from build123d import *

# Parameters (mm, degrees)
CHAMFER_SIZE    = 1
SKETCH001_R     = 2.25
SKETCH001_R_2   = 1.95
POCKET_DEPTH    = 2
CHAMFER001_SIZE = 0.5
POCKET001_DEPTH = 3


with BuildPart() as part:
    # Sketch (on XZ_Plane of Origin) → Revolution (revolve)
    with BuildSketch(Plane.XZ):
        Polygon((0, 0), (29.6, 0), (29.6, 7.7), (23.5, 7.7), (23.5, 6.2), (0, 6.2), align=None)
    revolve(axis=Axis((0, 0, 0), (0, 0, 1)))

    # Chamfer
    chamfer_edges = [part.edges().sort_by_distance(p)[0] for p in [
        (-23.5, 0, 7.7),
    ]]
    chamfer(chamfer_edges, length=CHAMFER_SIZE)

    # Sketch001 (on XY_Plane of Origin) → Pocket (cut)
    with BuildSketch(Plane.XY):
        Circle(SKETCH001_R)
        with Locations((14, 0)):
            Circle(SKETCH001_R_2)
        with Locations((-14, 0)):
            Circle(SKETCH001_R_2)
    extrude(amount=POCKET_DEPTH, mode=Mode.SUBTRACT)

    # Chamfer001
    chamfer001_edges = [part.edges().sort_by_distance(p)[0] for p in [
        (-29.6, 0, 7.7),
        (-29.6, 0, 0),
    ]]
    chamfer(chamfer001_edges, length=CHAMFER001_SIZE)

    # Sketch002 (on XY_Plane of Origin) → Pocket001 (cut)
    with BuildSketch(Plane.XY):
        with BuildLine():
            ThreePointArc((2, -22.1), (0, -20.1), (-2, -22.1))
            Line((-2, -22.1), (-2, -31.1))
            ThreePointArc((-2, -31.1), (0, -33.1), (2, -31.1))
            Line((2, -22.1), (2, -31.1))
        make_face()
    extrude(amount=POCKET001_DEPTH, mode=Mode.SUBTRACT)


solid = part.part
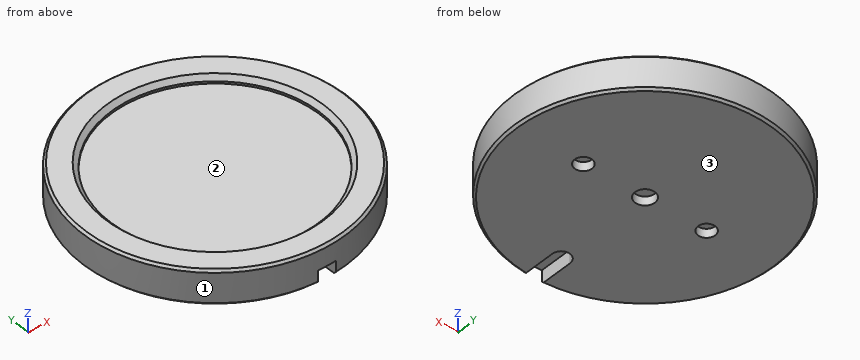
Geometry check sheet. Reference: the model listing, model coordinates, mm. Face numbers are marked on the shaded views. Round coordinates to 2 decimals unless told otherwise and drop trailing zeros. Write each loop counter-clockwise with the first axis right and the second up, starting at its lowest first coordinate (ties: lowest second). Pieces come first, ordered by that corner, then holes. Notation, with made-up numbers: (-1.5, 34.5) -> (54.5, 34.5) arc R16 cw to (54.5, 44.5) -> close; hole circle Ø4 at (-34.75, 4.25). An arc over 180 degrees is marked (long way). One line per item, written item: value. Start each with the question number.
(1) Cross-section at A-A, the plane y = 0. Record the cut outline in (x, z).
(2) Draft check along Y on the marked faces 1, 2 and 3. Enter one of: +Y half, -Y half, draft (parallel to the pull), parting line (faces both ways), or undercut.
(3) Cross-section at C-C, the plane z = 4. Record the cut outline in (x, y), and give its area (3 significant figures).
(4) Scan lines: line 1 (Y direction, x = 0, z = 0.75); line 2 (Y direction, x = 0, z = 6.4); line 3 (Z direction, x = -13.5, y = 0). Record each from-to range of solid material in increasing order. Write a range as [from, to].
(5) Go/stop test with flat-tipped pins: pin 1 Ø1 at (x, y) = (3, 11) entering from +Z; pin 2 Ø2 at (x, z) = (-16, 6) entering from -Y; pin 3 Ø4 at (y, z) = (-6, 5) entering from +X. Record where each tip stops, or that it passes through.
(6) Cross-section at B-B, the plane x = 0. Record the cut outline in (y, z), and give its area (3 significant figures).
Answer:
1. outline: (-29.6, 0.5) -> (-29.1, 0) -> (-15.95, 0) -> (-15.95, 2) -> (-12.05, 2) -> (-12.05, 0) -> (-2.25, 0) -> (-2.25, 2) -> (2.25, 2) -> (2.25, 0) -> (12.05, 0) -> (12.05, 2) -> (15.95, 2) -> (15.95, 0) -> (29.1, 0) -> (29.6, 0.5) -> (29.6, 7.2) -> (29.1, 7.7) -> (24.5, 7.7) -> (23.5, 6.7) -> (23.5, 6.2) -> (-23.5, 6.2) -> (-23.5, 6.7) -> (-24.5, 7.7) -> (-29.1, 7.7) -> (-29.6, 7.2) -> close
2. face 1: parting line
2. face 2: undercut
2. face 3: draft
3. outline: circle Ø59.2 at (0, 0)
3. area: 2,750 mm²
4. line 1: [-20.1, -2.25], [2.25, 29.6]
4. line 2: [-29.6, -23.5], [23.5, 29.6]
4. line 3: [2, 6.2]
5. pin 1: z = 6.2
5. pin 2: y = -25.52
5. pin 3: x = 29.33
6. outline: (-29.6, 3) -> (-20.1, 3) -> (-20.1, 0) -> (-2.25, 0) -> (-2.25, 2) -> (2.25, 2) -> (2.25, 0) -> (29.1, 0) -> (29.6, 0.5) -> (29.6, 7.2) -> (29.1, 7.7) -> (24.5, 7.7) -> (23.5, 6.7) -> (23.5, 6.2) -> (-23.5, 6.2) -> (-23.5, 6.7) -> (-24.5, 7.7) -> (-29.1, 7.7) -> (-29.6, 7.2) -> close
6. area: 346 mm²
